from build123d import *

# Parameters (mm, degrees)
SKETCH2_W           = 34
SKETCH2_H           = 60
BOSS_EXTRUDE1_DEPTH = 6
SKETCH3_R           = 1.5
CUT_EXTRUDE1_DEPTH  = 70.2242732
CHAMFER1_SIZE       = 2


with BuildPart() as part:
    # Sketch2 → Boss-Extrude1 (new body)
    with BuildSketch(Plane.XY):
        with Locations((17, 30)):
            Rectangle(SKETCH2_W, SKETCH2_H)
    extrude(amount=BOSS_EXTRUDE1_DEPTH)

    # Sketch3 → Cut-Extrude1 (cut, through all)
    with BuildSketch(Plane.XY.offset(6)):
        with Locations((3.75, 57)):
            Circle(SKETCH3_R)
        with Locations((30.25, 57)):
            Circle(SKETCH3_R)
        with Locations((3.75, 3)):
            Circle(SKETCH3_R)
        with Locations((30.25, 3)):
            Circle(SKETCH3_R)
    extrude(amount=-CUT_EXTRUDE1_DEPTH, mode=Mode.SUBTRACT)

    # Chamfer1
    chamfer1_edges = [part.edges().sort_by_distance(p)[0] for p in [
        (0, 60, 3),
        (34, 60, 3),
        (34, 0, 3),
        (0, 0, 3),
    ]]
    chamfer(chamfer1_edges, length=CHAMFER1_SIZE)


solid = part.part
CAD build for the part. Positions are in the model's coordinates, mm. Round coordinates to 2 decimals unless told otherwise and drop trailing zeros. Order: outer loops, then holes, each group sorted by start corner. A loop starts at its lowest first (then second) coordinate and runs counter-clockwise, first axis right, second up. Notation, with made-up numbers: (-33, -24) -> (2, -24) arc R35 cw to (2, 15) -> close; hole circle Ø6 at (81.5, 82.25). An arc over 180 degrees is marked (long way). Write each question's results on one line, items separated by ' | '.
1. Cut at C-C (z = 2.45). Give the cut face in (x, y).
Findings below:
outline: (0, 2) -> (2, 0) -> (32, 0) -> (34, 2) -> (34, 58) -> (32, 60) -> (2, 60) -> (0, 58) -> close; hole circle Ø3 at (3.75, 3); hole circle Ø3 at (3.75, 57); hole circle Ø3 at (30.25, 3); hole circle Ø3 at (30.25, 57)
2. Cut at A-A (y = 3). Give the cut face in (x, z), plus the area to 3 significant figures.
Findings below:
outline: (0, 0) -> (2.25, 0) -> (2.25, 6) -> (0, 6) -> close; (5.25, 0) -> (28.75, 0) -> (28.75, 6) -> (5.25, 6) -> close; (31.75, 0) -> (34, 0) -> (34, 6) -> (31.75, 6) -> close | area: 168 mm²
3. Wall check: line 1 along Y through (x, z) = (3.75, 1.4); line 2 along X through (y, z) = (56.5, 0.95); line 3 along Y through (x, z) = (29.5, 0.95). Give the ranges that are in metal, low to high. Write a range as [from, to].
Findings below:
line 1: y = [0, 1.5], [4.5, 55.5], [58.5, 60] | line 2: x = [0, 2.34], [5.16, 28.84], [31.66, 34] | line 3: y = [0, 1.7], [4.3, 55.7], [58.3, 60]
4. Cut at B-B (x = 30.25). Give the cut face in (y, z), plus the area to 3 significant figures.
Findings below:
outline: (0, 0) -> (1.5, 0) -> (1.5, 6) -> (0, 6) -> close; (4.5, 0) -> (55.5, 0) -> (55.5, 6) -> (4.5, 6) -> close; (58.5, 0) -> (60, 0) -> (60, 6) -> (58.5, 6) -> close | area: 324 mm²
5. Pull direction X, two halves, no side cores. Call faces 1 (the face through (34, 30, 3)), 2 (the face through (28.75, 3.07, 3.04)), 3 (the face through (1, 1, 3)), 4 (the face through (29.14, 58.01, 3.04)): pulls with the +X half, pulls with the -X half, needs draft (parallel to the pull), parting line crosses it, or undercut.
Findings below:
face 1: pulls with the +X half | face 2: undercut | face 3: pulls with the -X half | face 4: undercut
